CAD build for the part. Positions are in the model's coordinates, mm. A direction names the side the tool comes from. Coordinates: 2 decimals unless noted, no trailing zeros. Write each loop counter-clockwise with the first axis right and the second up, starting at its lowest first coordinate (ties: lowest second). Pieces come first, ordered by that corner, then holes. Notation, with made-up numbers: (-1.75, 15) -> (30.25, 15) arc R27 ccw to (30.25, 37) -> close; hole circle Ø7 at (9, -18.5). An arc over 180 degrees is marked (long way). Answer as CSV lines item,"result". Start each with the question number.
```python
from build123d import *

# Parameters (mm, degrees)
SKETCH1_W                 = 59.5
SKETCH1_H                 = 48
BOSS_EXTRUDE1_DEPTH       = 5
SKETCH2_W                 = 10
SKETCH2_H                 = 48
BOSS_EXTRUDE2_DEPTH       = 72.5
SKETCH3_W                 = 48
SKETCH3_H                 = 10
BOSS_EXTRUDE3_DEPTH       = 30
FILLET1_R                 = 10
F_1_0MM_START             = -72.5
F_1_0MM_DOWEL_SLOT1_DEPTH = 10
FILLET2_R                 = 10
M3_CLEARANCE_HOLE1_D      = 3.2
M6_CLEARANCE_HOLE1_D      = 6.4
CHAMFER1_SIZE             = 5


# Read off the part's stored shape, not the designer's step: Ø1.0mm Dowel Slot1
with BuildPart() as part:
    # Sketch1 → Boss-Extrude1 (new body)
    with BuildSketch(Plane(origin=(0, 0, 0), x_dir=(1, 0, 0), z_dir=(0, 1, 0))):
        with Locations((5.75, 0)):
            Rectangle(SKETCH1_W, SKETCH1_H)
    extrude(amount=BOSS_EXTRUDE1_DEPTH)

    # Sketch2 → Boss-Extrude2 (add)
    with BuildSketch(Plane.XZ):
        with Locations((30.5, 0)):
            Rectangle(SKETCH2_W, SKETCH2_H)
    extrude(amount=BOSS_EXTRUDE2_DEPTH)

    # Sketch3 → Boss-Extrude3 (add)
    with BuildSketch(Plane(origin=(35.5, 0, 0), x_dir=(0, 0, -1), z_dir=(1, 0, 0))):
        with Locations((0, -67.5)):
            Rectangle(SKETCH3_W, SKETCH3_H)
    extrude(amount=BOSS_EXTRUDE3_DEPTH)

    # Fillet1
    fillet1_edges = [part.edges().sort_by_distance(p)[0] for p in [
        (-24, 2.5, -24),
        (-24, 2.5, 24),
    ]]
    fillet(fillet1_edges, radius=FILLET1_R)

    # Ø1.0mm Dowel Slot1 outline → Ø1.0mm Dowel Slot1 (cut)
    with BuildSketch(Plane(origin=(0, 0, 0), x_dir=(1, 0, 0), z_dir=(0, 1, 0)).offset(F_1_0MM_START)):
        with BuildLine():
            Line((53, 14.75), (48, 14.75))
            ThreePointArc((48, 14.75), (45.25, 12), (48, 9.25))
            Line((48, 9.25), (53, 9.25))
            ThreePointArc((53, 9.25), (55.75, 12), (53, 14.75))
        make_face()
        with BuildLine():
            Line((53, -9.25), (48, -9.25))
            ThreePointArc((48, -9.25), (45.25, -12), (48, -14.75))
            Line((48, -14.75), (53, -14.75))
            ThreePointArc((53, -14.75), (55.75, -12), (53, -9.25))
        make_face()
    extrude(amount=F_1_0MM_DOWEL_SLOT1_DEPTH, mode=Mode.SUBTRACT)

    # Fillet2
    fillet2_edges = [part.edges().sort_by_distance(p)[0] for p in [
        (65.5, -67.5, 24),
        (65.5, -67.5, -24),
    ]]
    fillet(fillet2_edges, radius=FILLET2_R)

    # M3 Clearance Hole1 (through all)
    with Locations(Plane(origin=(0, 5, 0), x_dir=(1, 0, 0), z_dir=(0, 1, 0))):
        with Locations((-16.85, -9), (-16.85, 9), (16.15, 9), (16.15, -9)):
            Hole(M3_CLEARANCE_HOLE1_D / 2)

    # M6 Clearance Hole1 (through all)
    with Locations(Plane(origin=(0, 5, 0), x_dir=(1, 0, 0), z_dir=(0, 1, 0))):
        with Locations((-7.85, 0)):
            Hole(M6_CLEARANCE_HOLE1_D / 2)

    # Chamfer1
    chamfer1_edges = [part.edges().sort_by_distance(p)[0] for p in [
        (25.5, 0, 0),
        (35.5, -62.5, 0),
    ]]
    chamfer(chamfer1_edges, length=CHAMFER1_SIZE)


solid = part.part
```
1. Cut at D-D (z = -19). Give the cut face in (x, y).
2. Cut at A-A (x = -7.85). Give the cut face in (y, z).
3. Wall check: line 1 (X direction, y = 1.4, z = -9); line 2 (Z direction, x = 16.15, y = 1.5); line 3 (Z direction, x = -16.85, y = 2.85). Give the ranges that are in metal, low to high.
4. Tool access for faces 4 (the face through (25.5, -38, 0)), 5 (the face through (50, -68, -9.25)), 6 (the face through (53, -62.5, 0)), 7 (the face through (-24, 2, 0)): list every direction of +Z, -Z, +X, -X, +Y, -Y with a clear straight run to the whole face (end or side of a thin tool).
5. Mould opens along Z. For faces 1 (the face through (62.49, -67.43, 21.15)), 2 (the face through (55.75, -67.57, -11.94)), 3 (the face through (38, -60, 0)) say: pulls with the +Z half, pulls with the -Z half, needs draft (parallel to the pull), parting line crosses it, or undercut.
6. Cut at C-C (x = 16.15). Give the cut face in (y, z), then the cut area to 3 significant figures.
7. Cut at B-B (z = 0). Give the cut face in (x, y).
8. Flat gauge pins, fed straight in: P1, Ø6, axis at x = -4, z = 18.5, coming from the -Y side; P2, Ø20, axis at x = 52, z = 0.5, coming from the +Y side; P3, Ø3, axis at x = 16.15, z = 9, coming from the +Y side; P4, Ø5, axis at y = -40.5, z = -0.5, coming from the -X side. Where does each tip first touch, or does it go through?
Geometry check:
1,outline,"(-22.66, 0) -> (20.5, 0) -> (25.5, -5) -> (25.5, -72.5) -> (64.16, -72.5) -> (64.16, -62.5) -> (40.5, -62.5) -> (35.5, -57.5) -> (35.5, 5) -> (-22.66, 5) -> close"
2,outline,"(0, -24) -> (5, -24) -> (5, -3.2) -> (0, -3.2) -> close; (0, 3.2) -> (5, 3.2) -> (5, 24) -> (0, 24) -> close"
3,line 1,"-24 to -18.45, -15.25 to 14.55, 17.75 to 35.5"
3,line 2,"-24 to -10.6, -7.4 to 7.4, 10.6 to 24"
3,line 3,"-23.59 to -10.6, -7.4 to 7.4, 10.6 to 23.59"
4,face 4,"+Z, -Z, -X, -Y"
4,face 5,"+Y, -Y"
4,face 6,"+Z, -Z, +X, +Y"
4,face 7,"+Z, -Z, -X, +Y, -Y"
5,face 1,"pulls with the +Z half"
5,face 2,"undercut"
5,face 3,"needs draft"
6,outline,"(0, -24) -> (5, -24) -> (5, -10.6) -> (0, -10.6) -> close; (0, -7.4) -> (5, -7.4) -> (5, 7.4) -> (0, 7.4) -> close; (0, 10.6) -> (5, 10.6) -> (5, 24) -> (0, 24) -> close"
6,area,"208 mm²"
7,outline,"(-24, 0) -> (-11.05, 0) -> (-11.05, 5) -> (-24, 5) -> close; (-4.65, 0) -> (20.5, 0) -> (25.5, -5) -> (25.5, -72.5) -> (65.5, -72.5) -> (65.5, -62.5) -> (40.5, -62.5) -> (35.5, -57.5) -> (35.5, 5) -> (-4.65, 5) -> close"
8,P1,"y = 0"
8,P2,"y = -62.5"
8,P3,"through"
8,P4,"x = 25.5"
